Could you check a few things on this model? Use its own coordinates, in mm. A direction names the side the tool comes from. Coordinates: 2 decimals unless noted, no trailing zeros. Write each loop counter-clockwise with the first axis right and the second up, starting at its lowest first coordinate (ties: lowest second). Pieces come first, ordered by that corner, then holes. Notation, with made-up numbers: M 1,87 L 48,87 A22 cw 48,111 Z; hole C -10.75,0.25 d3. An arc over 180 degrees is marked long. Write item = value, one per line.
```python
from build123d import *

# Parameters (mm, degrees)
SKETCH1_W                                  = 74
SKETCH1_H                                  = 70
BOSS_EXTRUDE1_DEPTH                        = 47
SKETCH2_W                                  = 22.7
SKETCH2_H                                  = 19
CUT_EXTRUDE1_DEPTH                         = 68
SKETCH7_W                                  = 50
SKETCH7_H                                  = 23
CUT_EXTRUDE4_DEPTH                         = 50
SKETCH8_R                                  = 3.1
CUT_EXTRUDE5_DEPTH                         = 25
SKETCH9_W                                  = 20
SKETCH9_H                                  = 12
BOSS_EXTRUDE3_DEPTH                        = 20
SKETCH10_W                                 = 70
SKETCH10_H                                 = 12
BOSS_EXTRUDE4_DEPTH                        = 20
SKETCH12_R                                 = 3.5
CUT_EXTRUDE6_DEPTH                         = 20
MIRROR1_AT_THE_SECOND_PLANE_COPY_1_SKETC_R = 3.5
MIRROR1_AT_THE_SECOND_PLANE_COPY_1_DEPTH   = 20
SKETCH13_R                                 = 5.5
CUT_EXTRUDE7_DEPTH                         = 5
SKETCH14_R                                 = 3
CUT_EXTRUDE8_DEPTH                         = 10
SKETCH15_W                                 = 12.7
SKETCH15_H                                 = 5
CUT_EXTRUDE9_DEPTH                         = 20
SKETCH16_R                                 = 2
CUT_EXTRUDE10_DEPTH                        = 73.512067961


with BuildPart() as part:
    # Sketch1 → Boss-Extrude1 (new body)
    with BuildSketch(Plane(origin=(0, 0, 0), x_dir=(1, 0, 0), z_dir=(0, 1, 0))):
        Rectangle(SKETCH1_W, SKETCH1_H)
    extrude(amount=BOSS_EXTRUDE1_DEPTH)

    # Sketch2 → Cut-Extrude1 (cut)
    with BuildSketch(Plane(origin=(37, 0, 0), x_dir=(0, 0, -1), z_dir=(1, 0, 0))):
        with Locations((13.65, 37.5)):
            Rectangle(SKETCH2_W, SKETCH2_H)
    extrude(amount=-CUT_EXTRUDE1_DEPTH, mode=Mode.SUBTRACT)

    # Sketch7 → Cut-Extrude4 (cut)
    with BuildSketch(Plane(origin=(0, 0, -35), x_dir=(-1, 0, 0), z_dir=(0, 0, -1))):
        with Locations((-12, 11.5)):
            Rectangle(SKETCH7_W, SKETCH7_H)
    extrude(amount=-CUT_EXTRUDE4_DEPTH, mode=Mode.SUBTRACT)

    # Sketch8 → Cut-Extrude5 (cut)
    with BuildSketch(Plane.XY.offset(35)):
        with Locations((24.27, 22)):
            Circle(SKETCH8_R)
    extrude(amount=-CUT_EXTRUDE5_DEPTH, mode=Mode.SUBTRACT)

    # Sketch9 → Boss-Extrude3 (add)
    with BuildSketch(Plane(origin=(37, 0, 0), x_dir=(0, 0, -1), z_dir=(1, 0, 0))):
        with Locations((-25, 6)):
            Rectangle(SKETCH9_W, SKETCH9_H)
    extrude(amount=BOSS_EXTRUDE3_DEPTH)

    # Sketch10 → Boss-Extrude4 (add)
    with BuildSketch(Plane.ZY.offset(37)):
        with Locations((0, 6)):
            Rectangle(SKETCH10_W, SKETCH10_H)
    extrude(amount=BOSS_EXTRUDE4_DEPTH)

    # Sketch12 → Cut-Extrude6 (cut)
    with BuildSketch(Plane(origin=(0, 12, 0), x_dir=(1, 0, 0), z_dir=(0, 1, 0))):
        with Locations(Location((-47, 23, 0), (0, 0, 270))):
            Circle(SKETCH12_R)
    cut_extrude6 = extrude(amount=-CUT_EXTRUDE6_DEPTH, mode=Mode.SUBTRACT)

    # Mirror1: Cut-Extrude6 across plane
    add(cut_extrude6.mirror(Plane.XY), mode=Mode.SUBTRACT)

    # Mirror1 at the second plane: Cut-Extrude6 across plane
    add(cut_extrude6.mirror(Plane(origin=(0, 0, 0), x_dir=(0, 0, 1), z_dir=(1, 0, 0))), mode=Mode.SUBTRACT)

    # Mirror1 at the second plane copy 1 sketc → Mirror1 at the second plane copy 1 (cut)
    with BuildSketch(Plane(origin=(0, 12, 0), x_dir=(-1, 0, 0), z_dir=(0, 1, 0))):
        with Locations(Location((-47, 23, 0), (0, 0, 270))):
            Circle(MIRROR1_AT_THE_SECOND_PLANE_COPY_1_SKETC_R)
    extrude(amount=-MIRROR1_AT_THE_SECOND_PLANE_COPY_1_DEPTH, mode=Mode.SUBTRACT)

    # Sketch13 → Cut-Extrude7 (cut)
    with BuildSketch(Plane(origin=(0, 12, 0), x_dir=(1, 0, 0), z_dir=(0, 1, 0))):
        with Locations(Location((-47, -23, 0), (0, 0, 270))):
            Circle(SKETCH13_R)
    cut_extrude7 = extrude(amount=-CUT_EXTRUDE7_DEPTH, mode=Mode.SUBTRACT)

    # Mirror2: Cut-Extrude7 across plane
    add(cut_extrude7.mirror(Plane.XY), mode=Mode.SUBTRACT)

    # Mirror2 at the second plane: Cut-Extrude7 across plane
    add(cut_extrude7.mirror(Plane(origin=(0, 0, 0), x_dir=(0, 0, 1), z_dir=(1, 0, 0))), mode=Mode.SUBTRACT)

    # Sketch14 → Cut-Extrude8 (cut)
    with BuildSketch(Plane(origin=(-31, 0, 0), x_dir=(0, 0, -1), z_dir=(1, 0, 0))):
        with Locations((13.65, 37.5)):
            Circle(SKETCH14_R)
    extrude(amount=-CUT_EXTRUDE8_DEPTH, mode=Mode.SUBTRACT)

    # Sketch15 → Cut-Extrude9 (cut)
    with BuildSketch(Plane(origin=(37, 0, 0), x_dir=(0, 0, -1), z_dir=(1, 0, 0))):
        with Locations((13.65, 25.5)):
            Rectangle(SKETCH15_W, SKETCH15_H)
    extrude(amount=-CUT_EXTRUDE9_DEPTH, mode=Mode.SUBTRACT)

    # Sketch16 → Cut-Extrude10 (cut, through all)
    with BuildSketch(Plane(origin=(0, 28, 0), x_dir=(1, 0, 0), z_dir=(0, 1, 0))):
        with Locations(Location((4.53, 5.05, 0), (0, 0, 270))):
            Circle(SKETCH16_R)
        with Locations(Location((4.53, 22.25, 0), (0, 0, 270))):
            Circle(SKETCH16_R)
    extrude(amount=-CUT_EXTRUDE10_DEPTH, mode=Mode.SUBTRACT)


solid = part.part
```
Item 1: For faces 5 (the face through (41.547, 9.535, 22.284)), 6 (the face through (-13, 11, -10)), 7 (the face through (37, 33, 19)), 8 (the face through (-31, 40, -16)), which set-ups out of +Z, -Z, +X, -X, +Y, -Y let a thin tool reach every point of the face, with its end or its side?
Numbers:
face_5 = +Y
face_6 = -Z, +X, -Y
face_7 = +Z, -Z, +X, +Y
face_8 = +X, +Y
Item 2: Imagine slicing it at C-C (x = 47). Write out the boundary of the cut face in (y, z), and give its area (3 significant figures).
Numbers:
outline = M 0,15 L 12,15 L 12,17.5 L 7,17.5 L 7,19.5 L 0,19.5 Z; M 0,26.5 L 7,26.5 L 7,28.5 L 12,28.5 L 12,35 L 0,35 Z
area = 136 mm²
Item 3: Imagine slicing it at B-B (x = 4.53). Write out the boundary of the cut face in (y, z).
Numbers:
outline = M 0,15 L 23,15 L 23,-3.05 L 28,-3.05 L 28,-2.3 L 47,-2.3 L 47,35 L 0,35 Z; M 23,-35 L 47,-35 L 47,-25 L 28,-25 L 28,-24.25 L 23,-24.25 Z; M 23,-20.25 L 28,-20.25 L 28,-7.05 L 23,-7.05 Z
Item 4: If we mould it in two halves opening along Z, with no side actions, what happens to faces 1 (the face through (1, 18, 35)), 2 (the face through (-9, 28, -35)), 3 (the face through (17, 26, -14)), 4 (the face through (23.866, 25.074, 25.453))? For each: pulls with the +Z half, pulls with the -Z half, needs draft (parallel to the pull), parting line crosses it, or undercut.
Numbers:
face_1 = pulls with the +Z half
face_2 = pulls with the -Z half
face_3 = undercut
face_4 = needs draft
Item 5: I'm going to push flat-ended pins straight in: P1, Ø8, axis at x = 25.5, z = -9, coming from the -Y side; P2, Ø1, axis at x = -42, z = 0, coming from the +Y side; P3, Ø17.5, axis at x = 47, z = 23, coming from the -Y side; P4, Ø5.5, axis at y = 26, z = -16.5, coming from the +X side. Where does each tip first touch, or does it pass through?
Numbers:
P1 = 23
P2 = 12
P3 = 0
P4 = 17
Item 6: Imagine slicing it at A-A (z = -13.65). Write out the boundary of the cut face in (x, y).
Numbers:
outline = M -57,0 L -13,0 L -13,23 L 17,23 L 17,28 L -31,28 L -31,34.5 L -37,34.5 L -37,12 L -57,12 Z; M -37,40.5 L -31,40.5 L -31,47 L -37,47 Z
Item 7: If I drill on line 1 along X through (y, z) = (9.55, 23); line 2 along X through (y, z) = (4, 23); line 3 along Z through (x, y) = (28, 38), over which ranges is the centre line in solid material (lowest first)?
Numbers:
line_1 = -57 to -52.5, -41.5 to 41.5, 52.5 to 57
line_2 = -57 to -50.5, -43.5 to 43.5, 50.5 to 57
line_3 = -35 to -25, -2.3 to 35
Item 8: Imagine slicing it at D-D (y = 10). Write out the boundary of the cut face in (x, z), and give its area (3 significant figures).
Numbers:
outline = M -57,-35 L -13,-35 L -13,15 L 57,15 L 57,35 L -57,35 Z; hole C -47,-23 d11; hole C -47,23 d11; hole C 47,23 d11
area = 4,190 mm²
